Part model, mm, in its own coordinate system. Coordinates: 2 decimals unless noted, no trailing zeros. Loops run counter-clockwise (first coordinate to the right, second up) from the corner with the lowest first, then second, coordinate; pieces in that order, holes last. Notation, with made-up numbers: (20.5, 78) -> (39.5, 78) arc R34 cw to (39.5, 110) -> close; hole circle Ø9 at (-15.5, 22.5). An arc over 180 degrees is marked (long way). One line per item, written item: value. Start each with the question number.
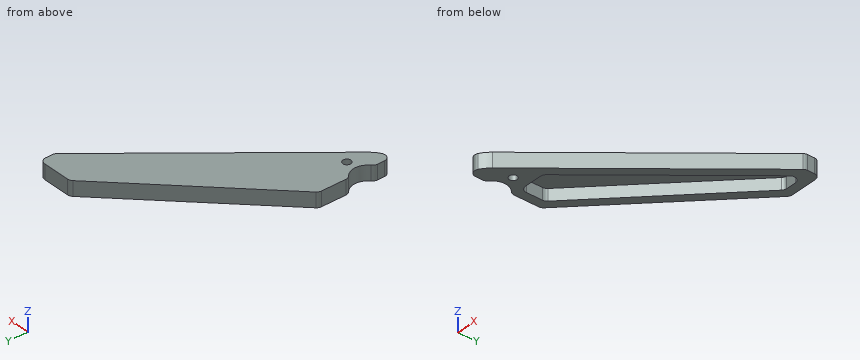
Autodesk Inventor part; units mm, degrees
ref_plane "YZ Plane" through (0, 0, 0) normal (1, 0, 0) x (0, 1, 0)
ref_plane "XZ Plane" through (0, 0, 0) normal (0, 1, 0) x (-1, 0, 0)
ref_plane "XY Plane" through (0, 0, 0) normal (0, 0, 1) x (1, 0, 0)
sketch "スケッチ1" plane through (0, 0, 0) normal (0, 0, 1) x (1, 0, 0)
  circle A0 centre (0, 0) radius 11 construction
  circle A1 centre (0, 8.5) radius 1.35
  circle A2 centre (0, 8.5) radius 2.5 construction
  circle A3 centre (0, 0) radius 5.05 construction
  circle A4 centre (0, -8.5) radius 1.35
  line L0 (48.7145, 60.75) -> (2.55, 14.5855)
  line L1 (0, 0) -> (0, 48.2635) construction
  line L2 (60.75, 60.75) -> (0, 0) construction
  line L3 (48.7145, 60.75) -> (60.75, 60.75)
  line L4 (60.75, 60.75) -> (60.75, 55.75)
  arc A5 (2.55, -10.7004) -> (8.4522, -7.0399) centre (0, 0) ccw
  line L5 (60.75, 55.75) -> (8.4522, -7.0399)
  circle A6 centre (0, 0) radius 8.5 construction
  circle A7 centre (8.5, 0) radius 1.35
  line L6 (2.55, 14.5855) -> (2.55, 4.3589)
  arc A8 (2.55, -4.3589) -> (2.55, 4.3589) centre (0, 0) ccw
  line L7 (2.55, -4.3589) -> (2.55, -10.7004)
  dimension "d3" = 10.1
  dimension "d0" = 2.7
  dimension "d1" = 8.5
  dimension "d2" = 5
  dimension "d6" = 360
  dimension "d11" = 45
  dimension "d13" = 60.75
  dimension "d17" = 5
  dimension "d18" = 2.55
extrude "押し出し1" add sketch "スケッチ1" along normal blind 5 contours L3 L4 L5 A5 L7 A8 L6 L0
fillet "フィレット1" radius 2 7 edges at (2.55, -10.7004, 2.5) (2.55, -4.3589, 2.5) (2.55, 14.5855, 2.5) (60.75, 60.75, 2.5) (60.75, 55.75, 2.5) (48.7145, 60.75, 2.5) (2.55, 4.3589, 2.5)
sketch "スケッチ2" plane through (0, 0, 0) normal (0, 0, -1) x (-1, 0, 0)
  line L0 (-2.55, 5.3852) -> (-2.55, 13.7571)
  line L1 (-3.1358, 15.1713) -> (-48.1287, 60.1642)
  line L2 (-49.5429, 60.75) -> (-58.75, 60.75)
  line L3 (-60.2868, 55.1938) -> (-8.4522, -7.0399)
  circle A0 centre (-8.5, 0) radius 1.35
  line L4 (-14.576, 5) -> (-58.5115, 57.75)
  line L5 (-58.5115, 57.75) -> (-49.9571, 57.75)
  line L6 (-49.9571, 57.75) -> (-5.55, 13.3429)
  line L7 (-5.55, 13.3429) -> (-5.55, 5)
  line L8 (-5.55, 5) -> (-14.576, 5)
  dimension "d20" = 5
  dimension "d21" = 3
  dimension "d22" = 3
  dimension "d23" = 3
  dimension "d24" = 3
extrude "押し出し2" cut sketch "スケッチ2" against normal blind 4 contours L4 L5 L6 L7 L8
fillet "フィレット2" radius 2 5 edges at (58.5115, 57.75, 2) (49.9571, 57.75, 2) (5.55, 5, 2) (14.576, 5, 2) (5.55, 13.3429, 2)
equation "\"d21\" = d22"
equation "\"d23\" = d22"
equation "\"d24\" = d23"
properties part number "頭_サブフレーム_1_1" material "アセタール樹脂、黒"
1) Slice it at C-C (x = 34.5). Give the cut face in (y, z).
2) Slice it at A-A (z = 2.45). Give the cut face in (x, y).
3) Slice it at B-B (y = 0). Give the cut face in (x, z), then the cut area to 3 significant figures.
4) Pin check, flat tips, straight feed: pin 1 Ø1.2 at (y, z) = (9.5, 1.5) entering from +X; pin 2 Ø1.2 at (x, z) = (10.5, 1) entering from +Y. Stop position of each tip, or through.
5) Probe line 1 (Y direction, x = 8.5, z = 2.3); line 2 (X direction, y = 23, z = 0.9); line 3 (Z direction, x = 8.5, y = 5.5). List the from-to ranges inside material, lowest first. Write a range as from..to.
6) Slice it at D-D (y = 25). Give the cut face in (x, z), then the cut area to 3 significant figures.
Check sheet entries:
1. outline: (24.23, 0) -> (28.92, 0) -> (28.92, 4) -> (42.29, 4) -> (42.29, 0) -> (46.54, 0) -> (46.54, 5) -> (24.23, 5) -> close
2. outline: (2.55, -7.77) arc R2 ccw to (5.56, -9.49) arc R11 ccw to (8.45, -7.04) -> (60.29, 55.19) arc R2 ccw to (60.75, 56.47) -> (60.75, 58.75) arc R2 ccw to (58.75, 60.75) -> (49.54, 60.75) arc R2 ccw to (48.13, 60.16) -> (3.14, 15.17) arc R2 ccw to (2.55, 13.76) -> (2.55, 5.39) arc R2 ccw to (3.26, 3.86) arc R5.05 cw to (3.26, -3.86) arc R2 ccw to (2.55, -5.39) -> close; hole (5.55, 7) arc R2 ccw to (7.55, 5) -> (13.64, 5) arc R2 ccw to (15.18, 5.72) -> (55.78, 54.47) arc R2 ccw to (54.24, 57.75) -> (50.79, 57.75) arc R2 ccw to (49.37, 57.16) -> (6.14, 13.93) arc R2 ccw to (5.55, 12.51) -> close; hole circle Ø2.7 at (8.5, 0)
3. outline: (5.05, 0) -> (7.15, 0) -> (7.15, 5) -> (5.05, 5) -> close; (9.85, 0) -> (14.32, 0) -> (14.32, 5) -> (9.85, 5) -> close
3. area: 32.8 mm^2
4. pin 1: stops at x = 22.73
4. pin 2: stops at y = 23.14
5. line 1: y = -6.98..-1.35, 1.35..5, 16.29..20.54
5. line 2: x = 10.96..15.21, 29.57..33.47
5. line 3: z = 4..5
6. outline: (12.96, 0) -> (17.21, 0) -> (17.21, 4) -> (31.23, 4) -> (31.23, 0) -> (35.14, 0) -> (35.14, 5) -> (12.96, 5) -> close
6. area: 54.8 mm^2
